Could you check a few things on this model? Use its own coordinates, in mm. A direction names the side the tool comes from. Give positions to 0.01 mm unless a question says otherwise; leave off trailing zeros. Write each loop counter-clockwise with the first axis right and the second up, starting at its lowest first coordinate (ties: lowest second). Pieces come first, ordered by that corner, then holes. Notation, with made-up numbers: (31.5, 66) - (37.5, 66) arc R28 ccw to (37.5, 97) - close; hole circle Ø2 at (51, -18.75). An arc over 180 degrees is marked (long way). Answer as CSV lines item,"result". Start each with the question number.
Q1. If I drill on line 1 along X through (y, z) = (-21.5, 5.25); line 2 along Y through (x, z) = (0, -1.3); line 3 along X through (y, z) = (33.5, 14.5), over which ranges is the centre line in solid material (lowest first)?
Q2. On a 3-axis mill with a long thin cutter (end or side, diameter ignored), from which of +Z, -Z, +X, -X, +Y, -Y can I reach the whole of each face in a straight line? I mean faces 4 (the face through (8.91, -36.174, 8.909)), 5 (the face through (12.569, -29.418, 7.464)), 6 (the face through (12.569, -30.015, 11.428)), 7 (the face through (8.91, 38.277, 15.367)). Say none if no direction works.
Q3. Imagine slicing it at C-C on x = 9.5. List the corners of the cut face in (y, z) for me (1 decimal), and give its area (3 significant figures).
Q4. Will these pins go through, and if not, where does the flat tip stop? pin 1 Ø1 at (x, y) = (12.5, 18.5) entering from -Z; pin 2 Ø1 at (x, z) = (-6, 1.5) entering from +Y; pin 3 Ø10 at (x, y) = (1, 16.5) entering from +Z; pin 4 Ø3 at (x, z) = (2, -2) entering from -Y.
Q5. We'd pull the mould along X, two halves only. Please class faces 1 (the face through (0, 0, -4)), 2 (the face through (16.09, -36.174, 8.909)), 3 (the face through (12.104, -34.595, 8.991)): pulls with the +X half, pulls with the -X half, needs draft (parallel to the pull), parting line crosses it, or undercut.
Q6. Imagine slicing it at D-D on z = 10. State how many separate pieces and enclosed holes the cut face has, and give its area (3 significant figures).
Q7. Imagine slicing it at A-A on y = 9.5. List the corners of the cut face in (x, z) for me, and give its area (3 significant figures).
Q8. Imagine slicing it at B-B on y = 0. List the corners of the cut face in (x, z) for me, and give its area (3 significant figures).
```python
from build123d import *

# Parameters (mm, degrees)
SKETCH1_W             = 34.925
SKETCH1_H             = 34.925
SKETCH1_R             = 1.6625
BOSS_EXTRUDE4_DEPTH   = 4
BOSS_EXTRUDE7_DEPTH   = 9.925
F_6_CLEARANCE_HOLE1_D = 3.6576
FILLET1_R             = 4.8125
FILLET2_R             = 2
FILLET1_OF_MIRROR1_R  = 4.8125
FILLET2_OF_MIRROR1_R  = 2


with BuildPart() as part:
    # Sketch1 → Boss-Extrude4 (new body)
    with BuildSketch(Plane.XY):
        Rectangle(SKETCH1_W, SKETCH1_H)
        with Locations((0, 9.5)):
            Circle(SKETCH1_R, mode=Mode.SUBTRACT)
        with Locations((9.5, 0)):
            Circle(SKETCH1_R, mode=Mode.SUBTRACT)
        with Locations((-9.5, 0)):
            Circle(SKETCH1_R, mode=Mode.SUBTRACT)
        with Locations((0, -9.5)):
            Circle(SKETCH1_R, mode=Mode.SUBTRACT)
    extrude(amount=-BOSS_EXTRUDE4_DEPTH)

    # Sketch7 → Boss-Extrude7 (add)
    with BuildSketch(Plane.ZY.offset(17.4625)):
        Polygon((0, 14.914218957), (11.825462524, 20.428522693), (16.011518882, 22.38051283), (17.512960324, 39.542067038), (13.528181531, 39.890690009), (12.228017656, 25.02974891), (-4, 17.4625), align=None)
        Polygon((8.02005001, -23.067541371), (6.762717001, -37.43892343), (10.747495793, -37.787546401), (12.248937235, -20.625992194), (8.391046827, -18.827028352), (0, -14.914218957), (-4, -17.4625), align=None)
    boss_extrude7 = extrude(amount=-BOSS_EXTRUDE7_DEPTH)

    # #6 Clearance Hole1 (through all)
    with Locations(Plane(origin=(0, -1.220180398, 13.946725773), x_dir=(1, 0, 0), z_dir=(0, -0.08715574274765159, 0.9961946980917462))):
        with Locations((-12.5, 36.1054526), (-12.5, -31.8945474)):
            f_6_clearance_hole1 = Hole(F_6_CLEARANCE_HOLE1_D / 2)

    # Fillet1
    fillet1_edges = [part.edges().sort_by_distance(p)[0] for p in [
        (-7.5375, -37.613234916, 8.755106397),
        (-17.4625, -37.613234916, 8.755106397),
        (-17.4625, 39.716378524, 15.520570928),
        (-7.5375, 39.716378524, 15.520570928),
    ]]
    fillet(fillet1_edges, radius=FILLET1_R)

    # Fillet2
    fillet2_edges = [part.edges().sort_by_distance(p)[0] for p in [
        (-12.5, -20.625992194, 12.248937235),
        (-12.5, -23.067541371, 8.02005001),
        (-12.5, -14.914218957, 0),
        (-12.5, 22.38051283, 16.011518882),
        (-12.5, 14.914218957, 0),
        (-12.5, 25.02974891, 12.228017656),
    ]]
    fillet(fillet2_edges, radius=FILLET2_R)

    # Mirror1: Boss-Extrude7, #6 Clearance Hole1 across plane
    add(boss_extrude7.mirror(Plane(origin=(0, 0, 0), x_dir=(0, 0, 1), z_dir=(1, 0, 0))))
    add(f_6_clearance_hole1.mirror(Plane(origin=(0, 0, 0), x_dir=(0, 0, 1), z_dir=(1, 0, 0))), mode=Mode.SUBTRACT)

    # Fillet1 of Mirror1
    fillet1_of_mirror1_edges = [part.edges().sort_by_distance(p)[0] for p in [
        (7.5375, -37.613234916, 8.755106397),
        (17.4625, -37.613234916, 8.755106397),
        (17.4625, 39.716378524, 15.520570928),
        (7.5375, 39.716378524, 15.520570928),
    ]]
    fillet(fillet1_of_mirror1_edges, radius=FILLET1_OF_MIRROR1_R)

    # Fillet2 of Mirror1
    fillet2_of_mirror1_edges = [part.edges().sort_by_distance(p)[0] for p in [
        (12.5, -20.625992194, 12.248937235),
        (12.5, -23.067541371, 8.02005001),
        (12.5, -14.914218957, 0),
        (12.5, 22.38051283, 16.011518882),
        (12.5, 14.914218957, 0),
        (12.5, 25.02974891, 12.228017656),
    ]]
    fillet(fillet2_of_mirror1_edges, radius=FILLET2_OF_MIRROR1_R)


solid = part.part
```
Conclusion:
1,line 1,"-17.46 to -7.54, 7.54 to 17.46"
1,line 2,"-17.46 to -11.16, -7.84 to 7.84, 11.16 to 17.46"
1,line 3,"-17.46 to -13.59, -11.41 to -7.54, 7.54 to 11.41, 13.59 to 17.46"
2,face 4,"-Z, -Y"
2,face 5,"-Z, +X, -X"
2,face 6,"+Z, +X, -X, -Y"
2,face 7,"+Z, +Y"
3,outline,"(-36.9, 10.8) - (-36.5, 6.8) - (-24.5, 7.9) arc R2 cw to (-22.5, 6.8) - (-17.5, -4) - (-1.7, -4) - (-1.7, 0) - (-13.6, 0) arc R2 cw to (-15.5, 1.2) - (-20, 11) arc R2 ccw to (-22, 12.1) - close; (1.7, -4) - (17.5, -4) - (24.5, 11.2) arc R2 cw to (26.2, 12.3) - (39, 13.4) - (38.6, 17.4) - (23.5, 16.1) arc R2 ccw to (21.9, 15) - (15.5, 1.2) arc R2 cw to (13.6, 0) - (1.7, 0) - close"
3,area,"362 mm^2"
4,pin 1,"z = -2.85"
4,pin 2,"through"
4,pin 3,"z = 0"
4,pin 4,"y = -17.46"
5,face 1,"needs draft"
5,face 2,"pulls with the +X half"
5,face 3,"undercut"
6,separate pieces,"4"
6,enclosed holes,"2"
6,area,"407 mm^2"
7,outline,"(-17.46, -4) - (-1.66, -4) - (-1.66, 0) - (-17.46, 0) - close; (1.66, -4) - (17.46, -4) - (17.46, 0) - (1.66, 0) - close"
7,area,"126 mm^2"
8,outline,"(-17.46, -4) - (-11.16, -4) - (-11.16, 0) - (-17.46, 0) - close; (-7.84, -4) - (7.84, -4) - (7.84, 0) - (-7.84, 0) - close; (11.16, -4) - (17.46, -4) - (17.46, 0) - (11.16, 0) - close"
8,area,"113 mm^2"
